Autodesk Inventor part; units mm, degrees
ref_plane "YZ Plane" through (0, 0, 0) normal (1, 0, 0) x (0, 1, 0)
ref_plane "XZ Plane" through (0, 0, 0) normal (0, 1, 0) x (-1, 0, 0)
ref_plane "XY Plane" through (0, 0, 0) normal (0, 0, 1) x (1, 0, 0)
sketch "Sketch2" plane through (0, 0, 0) normal (0, 0, 1) x (1, 0, 0)
  line L0 (0, 0) -> (-9.9, 0)
  line L1 (-9.9, 0) -> (-9.9, 105)
  line L2 (-9.9, 105) -> (0, 105)
  line L3 (0, 105) -> (0, 0)
  line L4 (-4.95, 0) -> (-4.95, 2.5)
  line L5 (-4.95, 0) -> (-2.45, 0) construction
  circle A0 centre (-4.95, 5) radius 2.5
  line L6 (-4.95, 7.5) -> (32.05, 7.5) construction
  line L7 (0, 44.5) -> (0, 0)
  line L8 (0, 0) -> (-9.9, 0)
  line L9 (-9.9, 0) -> (-9.9, 44.5)
  line L10 (0, 45.5) -> (0, 0)
  line L11 (0, 0) -> (-9.9, 0)
  line L12 (-9.9, 0) -> (-9.9, 45.5)
  line L13 (-4.95, 7.5) -> (66.05, 7.5) construction
  line L14 (-4.95, 7.5) -> (67.05, 7.5) construction
  line L15 (-9.9, 79.5) -> (0, 79.5)
  dimension "d35" = 5
  dimension "d4" = 9.9
  dimension "d5" = 105
  dimension "d33" = 2.5
  dimension "d34" = 90
extrude "Extrusion6" add sketch "Sketch2" along normal blind 5 contours L0 L1 L15 L3
properties part number "Cube_Holder_SB_V1_(71mm)"
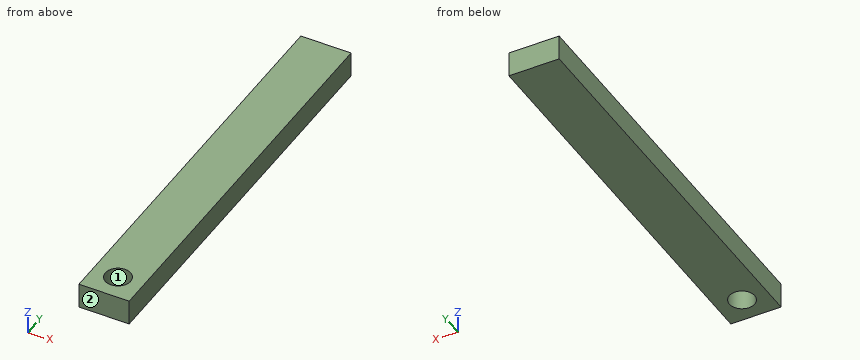
The listing builds one solid part. Answer for the finished solid, in the listing's coordinates (mm). Face numbers are marked on the shaded views. Give positions to 0.01 mm unless a question says otherwise; leave off trailing zeros. Order: outer loops, then holes, each group sorted by start corner. A loop starts at its lowest first (then second) coordinate and runs counter-clockwise, first axis right, second up. Notation, with made-up numbers: M -38.75,50 L 6.25,50 A25 ccw 6.25,89 Z; hole C -13,12.25 d3. An arc over 180 degrees is marked long. Put each result on its own line as item: value. Start each with the question number.
Item 1: Find the intervals of material crossed by line 1 along Y through (x, z) = (-4.95, 2.15); line 2 along X through (y, z) = (5, 3.15); line 3 along Y through (x, z) = (-3.25, 4.25), in increasing order.
Item 2: The part is cut by section C-C, the plane z = 2.45. Determine the outline of the cut face in (x, y).
Item 3: The part is cut by section B-B, the plane x = -4.95. Determine the outline of the cut face in (y, z).
Item 4: For a pull along X with two mould halves and no side action, classify the marked faces 1 and 2 as +X half, -X half, draft (parallel to the pull), parting line (faces both ways), or undercut.
Item 5: A flat-ended cylindrical pin translates along its axis: P1, Ø5, axis at x = -1.5, y = 38.5, coming from the -Z side. Find the tip coordinate at first contact, or state that the pin passes through.
Item 6: The part is cut by section A-A, the plane y = 5. Determine the outline of the cut face in (x, z), and give its area (3 significant figures).
Answer key:
1. line 1: y = 0 to 2.5, 7.5 to 79.5
1. line 2: x = -9.9 to -7.45, -2.45 to 0
1. line 3: y = 0 to 3.17, 6.83 to 79.5
2. outline: M -9.9,0 L 0,0 L 0,79.5 L -9.9,79.5 Z; hole C -4.95,5 d5
3. outline: M 0,0 L 2.5,0 L 2.5,5 L 0,5 Z; M 7.5,0 L 79.5,0 L 79.5,5 L 7.5,5 Z
4. face 1: undercut
4. face 2: draft
5. P1: stops at z = 0
6. outline: M -9.9,0 L -7.45,0 L -7.45,5 L -9.9,5 Z; M -2.45,0 L 0,0 L 0,5 L -2.45,5 Z
6. area: 24.5 mm²
